from build123d import *

# Parameters (mm, degrees)
SKETCH1_R                = 1.3
BOSS_EXTRUDE1_DEPTH      = 10
BOSS_EXTRUDE2_DEPTH      = 6
BOSS_EXTRUDE2_DEPTH_BACK = 2
SKETCH2_R                = 1.5
CHAMFER1_SIZE            = 0.2


with BuildPart() as part:
    # Sketch1 → Boss-Extrude1 (new body)
    with BuildSketch(Plane(origin=(0, 0, 0), x_dir=(1, 0, 0), z_dir=(0, 1, 0))):
        Polygon((-2.713546265, 0), (-1.356773133, -2.35), (1.356773133, -2.35), (2.713546265, 0), (1.356773133, 2.35), (-1.356773133, 2.35), align=None)
        with Locations(Location((0, 0, 0), (0, 0, 270))):
            Circle(SKETCH1_R, mode=Mode.SUBTRACT)
    extrude(amount=BOSS_EXTRUDE1_DEPTH)

    # Sketch2 → Boss-Extrude2 (add, two sides: drawn at the far end of the back side and taken through both)
    with BuildSketch(Plane.XZ.offset(-BOSS_EXTRUDE2_DEPTH_BACK)):
        with Locations(Location((0, 0, 0), (0, 0, 270))):
            Circle(SKETCH2_R)
    extrude(amount=BOSS_EXTRUDE2_DEPTH + BOSS_EXTRUDE2_DEPTH_BACK)

    # Chamfer1
    chamfer1_edges = [part.edges().sort_by_distance(p)[0] for p in [
        (0, -6, 1.5),
    ]]
    chamfer(chamfer1_edges, length=CHAMFER1_SIZE)

    # Sketch6 → Cut-Revolve1 (revolve, cut)
    with BuildSketch(Plane.XY, mode=Mode.PRIVATE) as cut_revolve1_sk:
        Polygon((-2.713546265, 10), (-2.713546265, 9.7), (-2.413546265, 10), align=None)
        Polygon((-2.413546265, 0), (-2.713546265, 0), (-2.713546265, 0.3), align=None)
    revolve(cut_revolve1_sk.sketch.rotate(Axis((0, 0, 0), (0, 1, 0)), 270), axis=Axis((0, 0, 0), (0, 1, 0)), mode=Mode.SUBTRACT)


solid = part.part
Geometry check sheet. Reference: the model listing, model coordinates, mm. A direction names the side the tool comes from. Give positions to 0.01 mm unless a question says otherwise; leave off trailing zeros. Loops run counter-clockwise (first coordinate to the right, second up) from the corner with the lowest first, then second, coordinate; pieces in that order, holes last. Notation, with made-up numbers: (-20.75, 84) -> (13.25, 84) arc R7 cw to (13.25, 89) -> close; hole circle Ø5 at (85, 26.5). An arc over 180 degrees is marked (long way). Answer in a Markdown table with one row per item. Add a question column.
1) Gauge pin test, flat end, axial feed: P1, Ø1.3, axis at x = 0, z = 0.5, coming from the +Y side. Record the tip position at first contact, or that the pin passes through.
2) Draft check along X on faces 1 (the face through (2.045, 4.93, -1.159)), 2 (the face through (1.039, 10, 1.012)), 3 (the face through (0.39, 5.94, 1.24)). Enter one of: pulls with the +X half, pulls with the -X half, needs draft (parallel to the pull), parting line crosses it, or undercut.
3) Cross-section at B-B on x = 0. Record the boundary of the cut face in (y, z), and give its area (3 significant figures).
4) Set-up check for faces 4 (the face through (0, 0, -2)), 5 (the face through (0, 2, 0)), 6 (the face through (0, 5, 2.35)): record each of +Z, -Z, +X, -X, +Y, -Y from which the full face is reachable in a straight line by a thin tool's end or side.
5) Material ranges on probe 1 along Z at (x, y) = (0, 8.75); probe 2 along Y at (x, z) = (2.2, 0.7); probe 3 along Y at (x, z) = (1.05, 0.1), recorded low to high. Write a range as from..to.
6) Cross-section at A-A on y = 5.5. Record the boundary of the cut face in (x, z).
Outcome:
| question | item | result |
|---|---|---|
| 1 | P1 | stops at y = 2 |
| 2 | face 1 | pulls with the +X half |
| 2 | face 2 | needs draft |
| 2 | face 3 | undercut |
| 3 | outline | (-6, -1.3) -> (-5.8, -1.5) -> (0, -1.5) -> (0, -2.35) -> (10, -2.35) -> (10, -1.3) -> (2, -1.3) -> (2, 1.3) -> (10, 1.3) -> (10, 2.35) -> (0, 2.35) -> (0, 1.5) -> (-5.8, 1.5) -> (-6, 1.3) -> close |
| 3 | area | 44.2 mm^2 |
| 4 | face 4 | -Y |
| 4 | face 5 | +Y |
| 4 | face 6 | +Z, +X, -X, +Y, -Y |
| 5 | probe 1 | z = -2.35..-1.3, 1.3..2.35 |
| 5 | probe 2 | y = 0..10 |
| 5 | probe 3 | y = -6..2 |
| 6 | outline | (-2.71, 0) -> (-1.36, -2.35) -> (1.36, -2.35) -> (2.71, 0) -> (1.36, 2.35) -> (-1.36, 2.35) -> close; hole circle Ø2.6 at (0, 0) |
